```python
from build123d import *

# Parameters (mm, degrees)
F0_W     = 50.8
F0_H     = 152.4
F1_DEPTH = 25.4
F2_R     = 5.08
F3_T     = -2.54


# Not quite as in the source:
# - a shell that OpenCascade refuses in one call is made with other operations: the cavity is built on its own and cut out


with BuildPart() as f1:
    # F0 (on Top) → F1 (new body)
    with BuildSketch(Plane.XY):
        Rectangle(F0_W, F0_H)
    extrude(amount=F1_DEPTH)

    # F2
    f2_edges = [f1.edges().sort_by_distance(p)[0] for p in [
        (-25.4, 76.2, 12.7),
        (25.4, 76.2, 12.7),
        (-25.4, -76.2, 12.7),
        (25.4, -76.2, 12.7),
        (25.4, 0, 25.4),
        (25.4, 0, 0),
        (-25.4, 0, 25.4),
        (-25.4, 0, 0),
    ]]
    fillet(f2_edges, radius=F2_R)

    # F3: a shell. OpenCascade refuses it in one call, so the cavity is built on its own and cut out:
    # the body offset inwards by the wall thickness, plus a prism from it out through each open face.
    f3_core = offset(f1.part, amount=F3_T, mode=Mode.PRIVATE)
    f3_exits = [f3_core.faces().sort_by_distance(p)[0] for p in [
        (-22.86, 0, 12.7),
    ]]
    add(f3_core, mode=Mode.SUBTRACT)
    extrude(f3_exits, amount=-F3_T, mode=Mode.SUBTRACT)


solid = f1.part
```
Design review of the part built by this model. Coordinates are the model's own, in mm. A direction names the side the tool comes from. Give positions to 0.01 mm unless a question says otherwise; leave off trailing zeros. Order: outer loops, then holes, each group sorted by start corner. A loop starts at its lowest first (then second) coordinate and runs counter-clockwise, first axis right, second up. Notation, with made-up numbers: (46, -32.75) - (78, -32.75) arc R9 ccw to (78, -28.75) - close; hole circle Ø6 at (-26, 13). An arc over 180 degrees is marked (long way). Use a Markdown table: item, result. Add a question column.
(1) Clearance check with flat-ended pins moving along their axes: P1, Ø7.5, axis at y = 16, z = 10.5, coming from the -X side; P2, Ø1.3, axis at x = -24, z = 11.5, coming from the +Y side; P3, Ø0.8, axis at x = -24.5, y = 14.5, coming from the +Z side. State where each tip first meets the part, or that it passes through.
(2) Add section B-B on y = -30. Give the boundary of the cut face in (x, z), then the cut area to 3 significant figures.
(3) Add section A-A on x = -16. Give the boundary of the cut face in (y, z).
(4) Wall thickness on probe 1 along Z at (x, y) = (-2, 43.5); probe 2 along Y at (x, z) = (-13.5, 9); probe 3 along Z at (x, y) = (-23, -66.5): over which ranges is each line inside the solid? List them lowest first. Write a range as [from, to].
(5) Add section C-C on z = 9.25. Give the boundary of the cut face in (x, y), then the cut area to 3 significant figures.
(6) Mouldability with a two-part tool opening along Z and no side actions: class faces 4 (the face through (-23.951, 74.672, 12.878)), 5 (the face through (0, 73.66, 13)), 6 (the face through (22.136, 72.896, 12.842)), 7 (the face through (-23.951, 1.067, 1.528)) as +Z half, -Z half, draft (parallel to the pull), parting line (faces both ways), or undercut.
(7) Machinability: for faces 1 (the face through (23.951, 1.067, 1.528)), 2 (the face through (-22.136, -72.896, 12.842)), 3 (the face through (-24, 71.12, 13)), which of the approach directions +Z, -Z, +X, -X, +Y, -Y give a long, thin tool a straight path to every point of the face, cutting with its end or side? Answer none if there is none.
Report:
| question | item | result |
|---|---|---|
| 1 | P1 | stops at x = 22.86 |
| 1 | P2 | stops at y = 75.2 |
| 1 | P3 | stops at z = 23.71 |
| 2 | outline | (-25.4, 5.08) arc R5.08 ccw to (-20.32, 0) - (20.32, 0) arc R5.08 ccw to (25.4, 5.08) - (25.4, 20.32) arc R5.08 ccw to (20.32, 25.4) - (-20.32, 25.4) arc R5.08 ccw to (-25.4, 20.32) - (-22.86, 20.32) arc R2.54 cw to (-20.32, 22.86) - (20.32, 22.86) arc R2.54 cw to (22.86, 20.32) - (22.86, 5.08) arc R2.54 cw to (20.32, 2.54) - (-20.32, 2.54) arc R2.54 cw to (-22.86, 5.08) - close |
| 2 | area | 306 mm² |
| 3 | outline | (-76.2, 0) - (76.2, 0) - (76.2, 25.4) - (-76.2, 25.4) - close; hole (-73.66, 2.54) - (73.66, 2.54) - (73.66, 22.86) - (-73.66, 22.86) - close |
| 4 | probe 1 | z = [0, 2.54], [22.86, 25.4] |
| 4 | probe 2 | y = [-76.2, -73.66], [73.66, 76.2] |
| 4 | probe 3 | z = [0.76, 5.08], [20.32, 24.64] |
| 5 | outline | (-25.4, -71.12) arc R5.08 ccw to (-20.32, -76.2) - (20.32, -76.2) arc R5.08 ccw to (25.4, -71.12) - (25.4, 71.12) arc R5.08 ccw to (20.32, 76.2) - (-20.32, 76.2) arc R5.08 ccw to (-25.4, 71.12) - (-22.86, 71.12) arc R2.54 cw to (-20.32, 73.66) - (20.32, 73.66) arc R2.54 cw to (22.86, 71.12) - (22.86, -71.12) arc R2.54 cw to (20.32, -73.66) - (-20.32, -73.66) arc R2.54 cw to (-22.86, -71.12) - close |
| 5 | area | 629 mm² |
| 6 | face 4 | draft |
| 6 | face 5 | undercut |
| 6 | face 6 | undercut |
| 6 | face 7 | -Z half |
| 7 | face 1 | -Z, +X, +Y, -Y |
| 7 | face 2 | none |
| 7 | face 3 | -X |
